Verification items for this drawing (mm, ordinates from the low corner). A direction names the side the tool comes from. Round coordinates to 2 decimals unless told otherwise and drop trailing zeros. Order: outer loops, then holes, each group sorted by start corner. A loop starts at its lowest first (then second) coordinate and runs counter-clockwise, first axis right, second up. Notation, with made-up numbers: M -24,46 L 4,46 A20 cw 4,69 Z; hole C 77,-20.75 d4. An arc over 180 degrees is marked long. One line per item, written item: value. Start each with the question number.
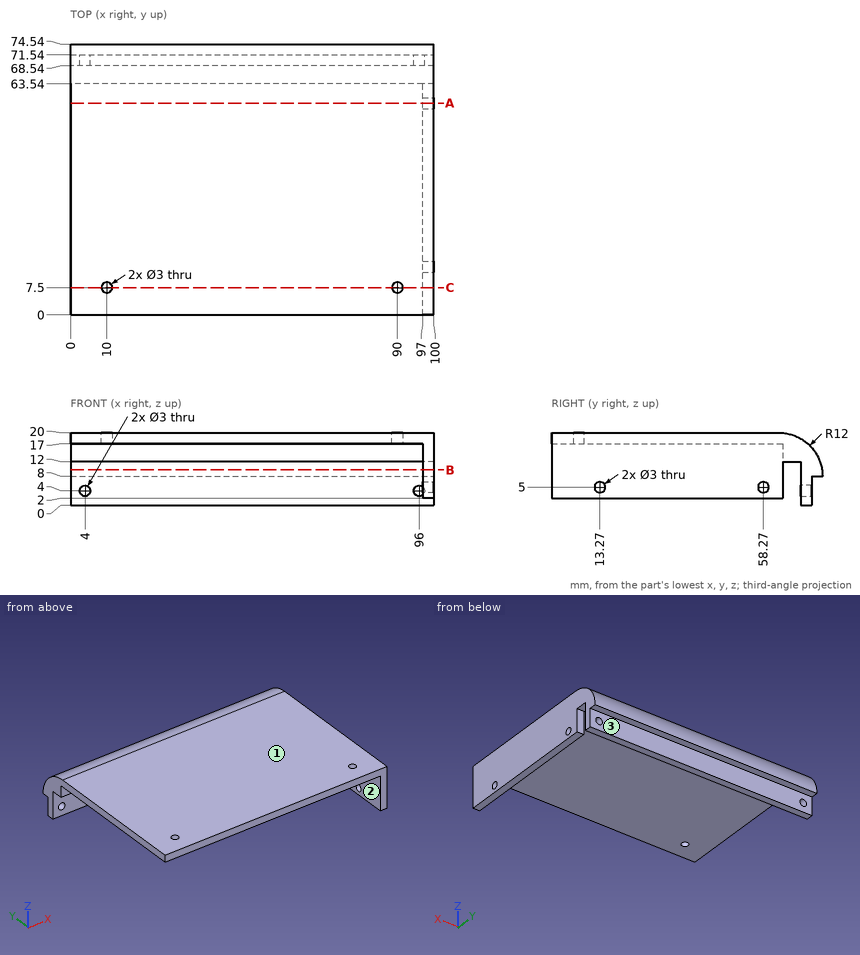
1. Section check A-A (y = 58.27). Record the cut outline in (x, z), and give its area (3 significant figures).
2. Section check B-B (z = 9.75). Record the cut outline in (x, y).
3. Scan lines: line 1 along Y through (x, z) = (98.7, 5); line 2 along X through (y, z) = (70.65, 4); line 3 along Z through (x, y) = (36, 54.5). Record each from-to range of solid material in increasing order.
4. Depth check by flat-ended pin: pin 1 (6 mm diameter, centred on x = 80.5, y = 34.5, fed in from -Z); pin 2 (4 mm diameter, centred on y = 34, z = 7, fed in from -X); pin 3 (2.5 mm diameter, centred on x = 50, y = 73, fed in from -Z); pin 4 (2.5 mm diameter, centred on y = 58.27, z = 5, fed in from +X). Enter the tip coordinate at first touch or a pass-through.
5. Section check C-C (y = 7.5). Record the cut outline in (x, z).
6. Tool access check on the marked faces 1, 2 and 3. Record the directions out of +Z, -Z, +X, -X, +Y, -Y that give a thin tool (end or side, any length) a straight path to the whole face; none if there is none.
Geometry check:
1. outline: M 0,17 L 97,17 L 97,6.5 L 100,6.5 L 100,20 L 0,20 Z; M 97,2 L 100,2 L 100,3.5 L 97,3.5 Z
1. area: 336 mm²
2. outline: M 0,68.54 L 100,68.54 L 100,74.41 L 0,74.41 Z; M 97,0 L 100,0 L 100,63.54 L 97,63.54 Z
3. line 1: y = 0 to 11.77, 14.77 to 56.77, 59.77 to 63.54, 68.54 to 71.54
3. line 2: x = 0 to 2.5, 5.5 to 94.5, 97.5 to 100
3. line 3: z = 17 to 20
4. pin 1: stops at z = 17
4. pin 2: stops at x = 97
4. pin 3: stops at z = 8
4. pin 4: passes through
5. outline: M 0,17 L 8.5,17 L 8.5,20 L 0,20 Z; M 11.5,17 L 88.5,17 L 88.5,20 L 11.5,20 Z; M 91.5,17 L 97,17 L 97,2 L 100,2 L 100,20 L 91.5,20 Z
6. face 1: +Z, +X, -X, +Y, -Y
6. face 2: -Z, -X, -Y
6. face 3: -Z, +X, -X, +Y
